The model under review builds one solid part; all positions refer to its coordinate system, in mm. Face numbers are marked on the shaded views. A direction names the side the tool comes from. Round coordinates to 2 decimals unless told otherwise and drop trailing zeros. Order: outer loops, then holes, each group sorted by start corner. A loop starts at its lowest first (then second) coordinate and runs counter-clockwise, first axis right, second up. Notation, with made-up numbers: M 53.25,22.25 L 95.25,22.25 A19 ccw 95.25,49.25 Z; hole C 65.5,51 d10. An arc over 180 degrees is marked long. Answer as a JSON object with one key per item and string values. Group by question number.
1) Consider section D-D, the plane y = -4. Write out the cut boundary in (x, z).
2) To check wall thickness, follow line 1 (Z direction, x = 10.65, y = 0); line 2 (Z direction, x = 5.25, y = 0); line 3 (Y direction, x = 11.2, z = 0). State the ranges of each line that lie inside material, in increasing order.
3) For the marked faces 1 and 2, list the 3-axis set-ups (+Z, -Z, +X, -X, +Y, -Y) from which the entire face can be reached by the end or side of a thin tool; tool diameter is ignored.
4) Insertion check: pin 1 Ø12 at (y, z) = (-1, 0) entering from -X; pin 2 Ø10 at (y, z) = (-5, 2) entering from -X; pin 3 Ø4 at (x, z) = (1.5, 4.5) entering from +Y; pin 4 Ø5 at (x, z) = (9.5, -3) entering from +Y. Each pin has a flat end and moves straight along its axis. Give the tip position at first contact, or say it passes through.
5) Consider section B-B, the plane z = 0. Write out the cut boundary in (x, y).
6) Consider section A-A, the plane y = 0. Write out the cut boundary in (x, z), then the cut area to 3 significant figures.
7) Consider section C-C, the plane x = 7.75. Write out the cut boundary in (y, z), then the cut area to 3 significant figures.
8) The part is to be moulded in two halves that separate along Z. For the marked faces 3, 4, 5 and 6, say which applies: +Z half, -Z half, draft (parallel to the pull), parting line (faces both ways), or undercut.
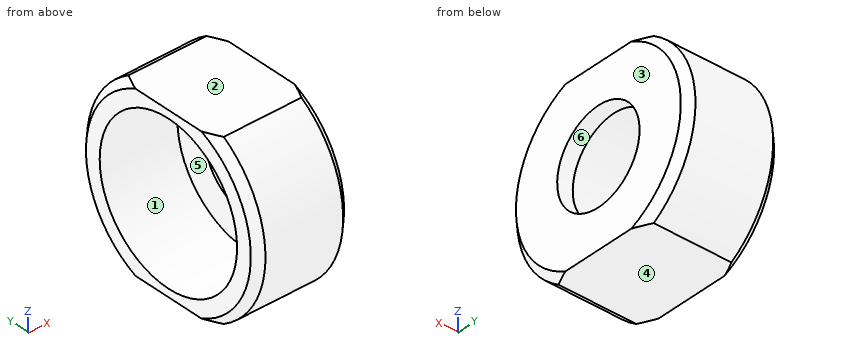
```python
from build123d import *

# Parameters (mm, degrees)
F2_SIZE  = 1
F3_W     = 15.3355175093
F3_H     = 4.7520212233
F3_W_2   = 15.3147058821
F3_H_2   = 7.7273081392
F4_DEPTH = 12.5


with BuildPart() as f1:
    # F0 (on Front) → F1 (revolve)
    with BuildSketch(Plane.XZ):
        Polygon((0, 13), (0, 10), (10, 10), (10, 6), (12, 6), (12, 13), align=None)
    revolve(axis=Axis((0.2130177937, 0, 0), (1, 0, 0)))

    # F2
    f2_edges = [f1.edges().sort_by_distance(p)[0] for p in [
        (12, 0, -13),
        (0, 0, -13),
    ]]
    chamfer(f2_edges, length=F2_SIZE)

    # F3 (on Front) → F4 (cut, symmetric)
    with BuildSketch(Plane.XZ):
        with Locations((7.1024957381, 13.3760106117)):
            Rectangle(F3_W, F3_H)
        with Locations((7.2143123355, -14.8636540696)):
            Rectangle(F3_W_2, F3_H_2)
    extrude(amount=F4_DEPTH, both=True, mode=Mode.SUBTRACT)


solid = f1.part
```
Results list:
{
 "1": {"outline": "M 0,-11 L 12,-11 L 12,-4.47 L 10,-4.47 L 10,-9.17 L 0,-9.17 Z; M 0,9.17 L 10,9.17 L 10,4.47 L 12,4.47 L 12,11 L 0,11 Z"},
 "2": {"line 1": "-11 to -6, 6 to 11", "line 2": "-11 to -10, 10 to 11", "line 3": "-12.8 to -6, 6 to 12.8"},
 "3": {"face 1": "-X", "face 2": "+Z, +X, -X, +Y, -Y"},
 "4": {"pin 1": "x = 10", "pin 2": "x = 0", "pin 3": "y = 12.76", "pin 4": "y = 12.99"},
 "5": {"outline": "M 0,-12 L 1,-13 L 11,-13 L 12,-12 L 12,-6 L 10,-6 L 10,-10 L 0,-10 Z; M 0,10 L 10,10 L 10,6 L 12,6 L 12,12 L 11,13 L 1,13 L 0,12 Z"},
 "6": {"outline": "M 0,-11 L 12,-11 L 12,-6 L 10,-6 L 10,-10 L 0,-10 Z; M 0,10 L 10,10 L 10,6 L 12,6 L 12,11 L 0,11 Z", "area": "40.0 mm^2"},
 "7": {"outline": "M -6.93,-11 L 6.93,-11 A13 ccw 6.93,11 L -6.93,11 A13 ccw Z; hole C 0,0 d20", "area": "179 mm^2"},
 "8": {"face 3": "draft", "face 4": "-Z half", "face 5": "undercut", "face 6": "undercut"}
}
